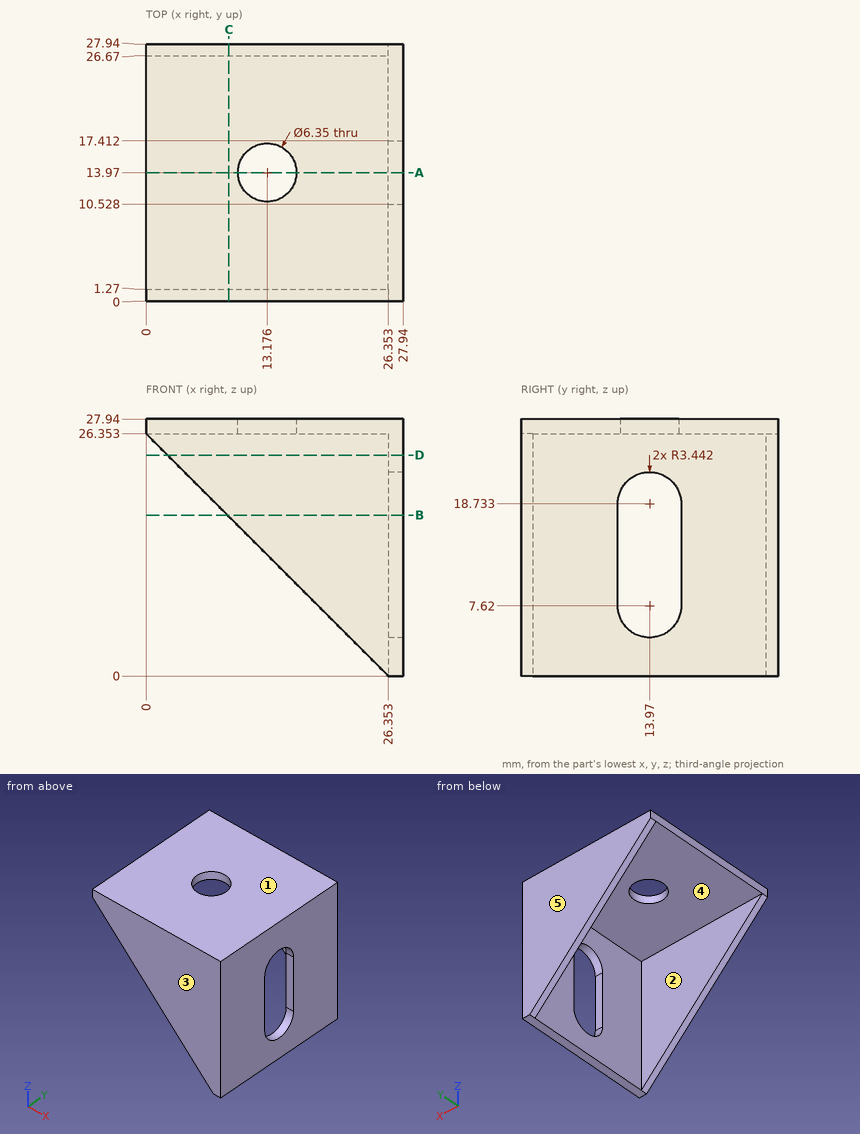
Part print with two shaded views. Sizes in mm from the minimum x, y, z corner. A direction names the side the tool comes from. Give positions to 0.01 mm unless a question says otherwise; leave off trailing zeros. Loops run counter-clockwise (first coordinate to the right, second up) from the corner with the lowest first, then second, coordinate; pieces in that order, holes last. Notation, with made-up numbers: (6, 46.25) - (14, 46.25) arc R17 ccw to (14, 53.25) - close; hole circle Ø4 at (-9.5, 28). An arc over 180 degrees is marked (long way). Put each result on its own line as item: value.
Q1. Slice it at B-B (z = 17.5). Give the cut face in (x, y).
Filled in:
outline: (8.85, 0) - (27.94, 0) - (27.94, 10.53) - (26.35, 10.53) - (26.35, 1.27) - (8.85, 1.27) - close; (8.85, 26.67) - (26.35, 26.67) - (26.35, 17.41) - (27.94, 17.41) - (27.94, 27.94) - (8.85, 27.94) - close
Q2. Mould opens along Y. For the marked faces 3, 4 and 5 say: pulls with the +Y half, pulls with the -Y half, needs draft (parallel to the pull), parting line crosses it, or undercut.
Filled in:
face 3: pulls with the -Y half
face 4: undercut
face 5: pulls with the +Y half
Q3. Probe line 1 along Y through (x, z) = (25, 20.5); line 2 along X through (y, z) = (22.5, 14.5). List the from-to ranges inside material, lowest first.
Filled in:
line 1: y = 0 to 1.27, 26.67 to 27.94
line 2: x = 26.35 to 27.94
Q4. Tool access for the marked faces 1 and 2: list every direction of +Z, -Z, +X, -X, +Y, -Y with a clear straight run to the whole face (end or side of a thin tool).
Filled in:
face 1: +Z, +X, -X, +Y, -Y
face 2: -Z, -X
Q5. Slice it at A-A (y = 13.97). Give the cut face in (x, z) (1 decimal).
Filled in:
outline: (0, 26.4) - (10, 26.4) - (10, 27.9) - (0, 27.9) - close; (16.4, 26.4) - (26.4, 26.4) - (26.4, 22.2) - (27.9, 22.2) - (27.9, 27.9) - (16.4, 27.9) - close; (26.4, 0) - (27.9, 0) - (27.9, 4.2) - (26.4, 4.2) - close
Q6. Slice it at D-D (z = 24). Give the cut face in (x, y).
Filled in:
outline: (2.35, 0) - (27.94, 0) - (27.94, 27.94) - (2.35, 27.94) - (2.35, 26.67) - (26.35, 26.67) - (26.35, 1.27) - (2.35, 1.27) - close
Q7. Flat gauge pins, fed straight in: pin 1 (12.5 mm diameter, centred on x = 8.5, y = 11, fed in from -Z); pin 2 (7.5 mm diameter, centred on y = 15.5, z = 6.5, fed in from -X). Where does each tip first touch, or does it go through?
Filled in:
pin 1: stops at z = 26.35
pin 2: stops at x = 26.35
Q8. Slice it at C-C (x = 9). Give the cut face in (y, z).
Filled in:
outline: (0, 17.35) - (1.27, 17.35) - (1.27, 26.35) - (26.67, 26.35) - (26.67, 17.35) - (27.94, 17.35) - (27.94, 27.94) - (0, 27.94) - close
